The model under review builds one solid part; all positions refer to its coordinate system, in mm. Round coordinates to 2 decimals unless told otherwise and drop trailing zeros. Order: outer loops, then holes, each group sorted by start corner. A loop starts at its lowest first (then second) coordinate and runs counter-clockwise, first axis right, second up. Notation, with made-up numbers: M 9.25,56 L 53.25,56 A18 cw 53.25,71 Z; hole C -9,-11 d2. An arc over 180 degrees is marked long. Use a Markdown table: item, result. Add a question column.
1. Consider section A-A on z = -74. State the section outline as (x, y) points.
2. To check wall thickness, follow probe 1 along Z at (x, y) = (10.5, 0.95); probe 2 along X at (y, z) = (1, -75); probe 3 along X at (y, z) = (1, -70). State the ranges of each line that lie inside material, in increasing order.
3. Consider section B-B on x = 12.7. State the section outline as (y, z) points.
4. Consider section C-C on y = 0.3. Count the separate pieces of the cut face and the enclosed holes in it, then the cut area to 3 significant figures.
5. Insertion check: P1, Ø0.5, axis at y = 1, z = 1.5, coming from the -X side (3 decimals); P2, Ø0.5, axis at y = 1, z = 1, coming from the +X side (3 decimals); P3, Ø0.5, axis at x = 15, y = 1, coming from the +Z side. Each pin has a flat end and moves straight along its axis. Give the tip position at first contact, or say it passes through.
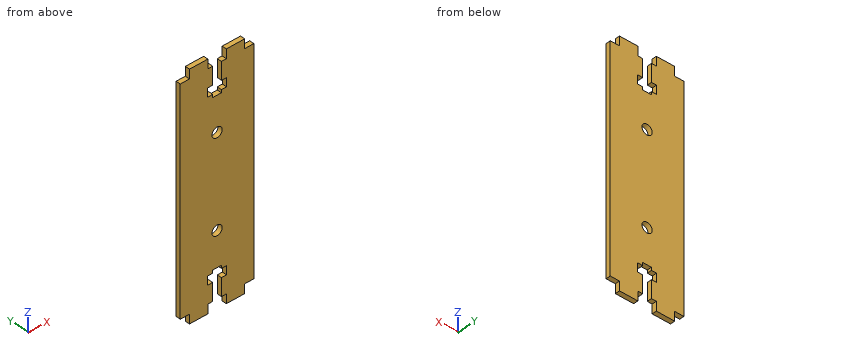
from build123d import *

# Parameters (mm, degrees)
SKETCH1_W           = 6.35
SKETCH1_H           = 3.175
BOSS_EXTRUDE1_DEPTH = 1.5875
SKETCH2_R           = 1.76403
CUT_EXTRUDE1_DEPTH  = 1.5875


with BuildPart() as part:
    # Sketch1 → Boss-Extrude1 (new body)
    with BuildSketch(Plane(origin=(0, 0, 0), x_dir=(1, 0, 0), z_dir=(0, 1, 0))):
        Polygon((0, 76.2), (0, 0), (3.175, 0), (9.525, 0), (11.2, 0), (11.2, 6.144), (9.45, 6.144), (9.45, 9.144), (11.2, 9.144), (11.2, 10.16), (14.2, 10.16), (14.2, 9.144), (15.95, 9.144), (15.95, 6.144), (14.2, 6.144), (14.2, 0), (15.875, 0), (22.225, 0), (25.4, 0), (25.4, 76.2), (22.225, 76.2), (15.875, 76.2), (14.2, 76.2), (14.2, 70.056), (15.95, 70.056), (15.95, 67.056), (14.2, 67.056), (14.2, 66.04), (11.2, 66.04), (11.2, 67.056), (9.45, 67.056), (9.45, 70.056), (11.2, 70.056), (11.2, 76.2), (9.525, 76.2), (3.175, 76.2), align=None)
        with Locations((6.35, 77.7875)):
            Rectangle(SKETCH1_W, SKETCH1_H)
        with Locations((19.05, 77.7875)):
            Rectangle(SKETCH1_W, SKETCH1_H)
        with Locations((6.35, -1.5875)):
            Rectangle(SKETCH1_W, SKETCH1_H)
        with Locations((19.05, -1.5875)):
            Rectangle(SKETCH1_W, SKETCH1_H)
    extrude(amount=BOSS_EXTRUDE1_DEPTH)

    # Sketch2 → Cut-Extrude1 (cut)
    with BuildSketch(Plane(origin=(0, 1.5875, 0), x_dir=(1, 0, 0), z_dir=(0, 1, 0))):
        with Locations(Location((12.7, 53.975, 0), (0, 0, 270))):
            Circle(SKETCH2_R)
        with Locations(Location((12.7, 22.225, 0), (0, 0, 270))):
            Circle(SKETCH2_R)
    extrude(amount=-CUT_EXTRUDE1_DEPTH, mode=Mode.SUBTRACT)


solid = part.part
Answer block:
| question | item | result |
|---|---|---|
| 1 | outline | M 0,0 L 11.2,0 L 11.2,1.59 L 0,1.59 Z; M 14.2,0 L 25.4,0 L 25.4,1.59 L 14.2,1.59 Z |
| 2 | probe 1 | -76.2 to -70.06, -67.06 to -9.14, -6.14 to 0 |
| 2 | probe 2 | 0 to 11.2, 14.2 to 25.4 |
| 2 | probe 3 | 0 to 9.45, 15.95 to 25.4 |
| 3 | outline | M 0,-66.04 L 1.59,-66.04 L 1.59,-55.74 L 0,-55.74 Z; M 0,-52.21 L 1.59,-52.21 L 1.59,-23.99 L 0,-23.99 Z; M 0,-20.46 L 1.59,-20.46 L 1.59,-10.16 L 0,-10.16 Z |
| 4 | separate pieces | 1 |
| 4 | enclosed holes | 2 |
| 4 | area | 1,910 mm^2 |
| 5 | P1 | x = 3.175 |
| 5 | P2 | x = 22.225 |
| 5 | P3 | z = 0 |
